Here's how the part is built. I have some questions about the finished solid (model axes, mm). Round coordinates to 2 decimals unless told otherwise and drop trailing zeros. Order: outer loops, then holes, each group sorted by start corner. A loop starts at its lowest first (then second) coordinate and runs counter-clockwise, first axis right, second up. Notation, with made-up numbers: (-1.5, 58.5) - (11.5, 58.5) arc R31 ccw to (11.5, 97.5) - close; hole circle Ø11 at (5.5, -17.75). An arc over 180 degrees is marked (long way). Answer as a JSON object with one key per item and string values.
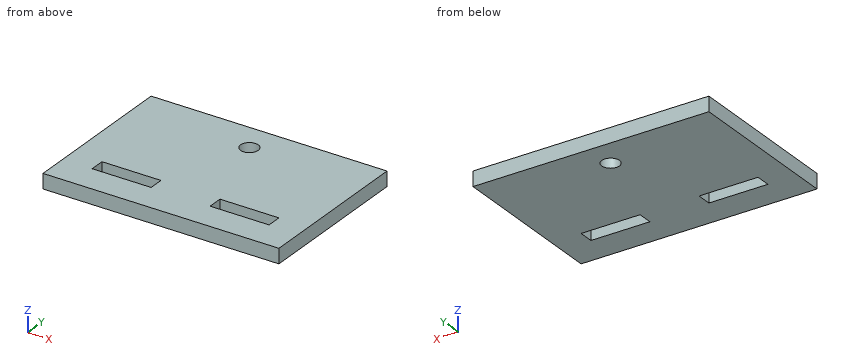
```python
from build123d import *

# Parameters (mm, degrees)
SKETCH1_W           = 50.8
SKETCH1_H           = 34.925
SKETCH1_R           = 1.905
SKETCH1_W_2         = 12.7
SKETCH1_H_2         = 3.175
BOSS_EXTRUDE1_DEPTH = 3.175


with BuildPart() as part:
    # Sketch1 → Boss-Extrude1 (new body)
    with BuildSketch(Plane.XY):
        with Locations((25.4, 17.4625)):
            Rectangle(SKETCH1_W, SKETCH1_H)
        with Locations((25.4, 28.575)):
            Circle(SKETCH1_R, mode=Mode.SUBTRACT)
        with Locations((12.7, 7.9375)):
            Rectangle(SKETCH1_W_2, SKETCH1_H_2, mode=Mode.SUBTRACT)
        with Locations((38.1, 7.9375)):
            Rectangle(SKETCH1_W_2, SKETCH1_H_2, mode=Mode.SUBTRACT)
    extrude(amount=BOSS_EXTRUDE1_DEPTH)


solid = part.part
```
1. Imagine slicing it at B-B (y = 7). List the corners of the cut face in (x, z) for me (3 decimals).
Responses:
{"outline": "(0, 0) - (6.35, 0) - (6.35, 3.175) - (0, 3.175) - close; (19.05, 0) - (31.75, 0) - (31.75, 3.175) - (19.05, 3.175) - close; (44.45, 0) - (50.8, 0) - (50.8, 3.175) - (44.45, 3.175) - close"}
2. For P1, Ø3, axis at x = 25.4, y = 28.575, coming from the -Z side, with a flat end and sliding along its axis, tell me the tip position at first contact or that it passes through.
Responses:
{"P1": "through"}
3. If I drill on L1, parallel to X at y = 9, z = 1.9; L2, parallel to Y at x = 6.5, z = 1.65 (3 decimals); L3, parallel to Y at x = 25.4, z = 1 (3 decimals), over which ranges is the centre line in solid material (lowest first)? Write a range as [from, to].
Responses:
{"L1": "[0, 6.35], [19.05, 31.75], [44.45, 50.8]", "L2": "[0, 6.35], [9.525, 34.925]", "L3": "[0, 26.67], [30.48, 34.925]"}
4. Imagine slicing it at A-A (x = 25.4). List the corners of the cut face in (y, z) for me (3 decimals).
Responses:
{"outline": "(0, 0) - (26.67, 0) - (26.67, 3.175) - (0, 3.175) - close; (30.48, 0) - (34.925, 0) - (34.925, 3.175) - (30.48, 3.175) - close"}
5. Imagine slicing it at C-C (z = 2.5). List the corners of the cut face in (x, y) for me (3 decimals).
Responses:
{"outline": "(0, 0) - (50.8, 0) - (50.8, 34.925) - (0, 34.925) - close; hole (6.35, 6.35) - (19.05, 6.35) - (19.05, 9.525) - (6.35, 9.525) - close; hole circle Ø3.81 at (25.4, 28.575); hole (31.75, 6.35) - (44.45, 6.35) - (44.45, 9.525) - (31.75, 9.525) - close"}
6. Imagine slicing it at D-D (x = 36). List the corners of the cut face in (y, z) for me (3 decimals).
Responses:
{"outline": "(0, 0) - (6.35, 0) - (6.35, 3.175) - (0, 3.175) - close; (9.525, 0) - (34.925, 0) - (34.925, 3.175) - (9.525, 3.175) - close"}
